```python
from build123d import *

# Parameters (mm, degrees)
SKETCH_1_W               = 135
SKETCH_1_H               = 100
EXTRUDE_1_DEPTH          = 4
SKETCH_2_W               = 135
SKETCH_2_H               = 4
EXTRUDE_2_DEPTH          = 60
CUT_EXTRUDE_1_DEPTH      = 130.12106722
CUT_EXTRUDE_1_DEPTH_BACK = 130.12106722
SKETCH_3_W               = 3
SKETCH_3_H               = 50
FILLET_1_R               = 5
FILLET_2_R               = 2
CUT_EXTRUDE_2_DEPTH      = 130.12106722
CUT_EXTRUDE_2_DEPTH_BACK = 130.12106722
SKETCH_4_R               = 1.75
CUT_EXTRUDE_3_DEPTH      = 130.12106722
CUT_EXTRUDE_3_DEPTH_BACK = 130.12106722
SKETCH_5_W               = 34
SKETCH_5_H               = 12
CUT_EXTRUDE_4_DEPTH      = 130.12106722
CUT_EXTRUDE_4_DEPTH_BACK = 130.12106722
SKETCH_6_R               = 1.75
CUT_EXTRUDE_5_DEPTH      = 130.12106722
CUT_EXTRUDE_5_DEPTH_BACK = 130.12106722
SKETCH_7_R               = 1.63491013
CUT_EXTRUDE_6_DEPTH      = 130.12106722
CUT_EXTRUDE_6_DEPTH_BACK = 130.12106722
SKETCH_8_R               = 1.5
SKETCH_9_R               = 1.75
EXTRUDE_3_DEPTH          = 3
CUT_EXTRUDE_7_DEPTH      = 130.12106722
CUT_EXTRUDE_7_DEPTH_BACK = 130.12106722
SKETCH_10_R              = 1.75


with BuildPart() as part:
    # 草图1 → 凸台-拉伸1 (new body)
    with BuildSketch(Plane(origin=(0, 0, 0), x_dir=(1, 0, 0), z_dir=(0, 1, 0))):
        Rectangle(SKETCH_1_W, SKETCH_1_H)
    extrude(amount=EXTRUDE_1_DEPTH)

    # 草图2 → 凸台-拉伸2 (add)
    with BuildSketch(Plane.XY.offset(50)):
        with Locations((0, 2)):
            Rectangle(SKETCH_2_W, SKETCH_2_H)
    extrude(amount=EXTRUDE_2_DEPTH)

    # 草图3 → 切除-拉伸1 (cut, two sides: drawn at the far end of the back side and taken through both)
    with BuildSketch(Plane(origin=(0, 4, 0), x_dir=(1, 0, 0), z_dir=(0, 1, 0)).offset(-CUT_EXTRUDE_1_DEPTH_BACK)):
        with Locations((-66, 25)):
            Rectangle(SKETCH_3_W, SKETCH_3_H)
        with Locations((66, 25)):
            Rectangle(SKETCH_3_W, SKETCH_3_H)
        with Locations((-66, -85)):
            Rectangle(SKETCH_3_W, SKETCH_3_H)
        with Locations((66, -85)):
            Rectangle(SKETCH_3_W, SKETCH_3_H)
    extrude(amount=CUT_EXTRUDE_1_DEPTH + CUT_EXTRUDE_1_DEPTH_BACK, mode=Mode.SUBTRACT)

    # 圆角1
    fillet_1_edges = [part.edges().sort_by_distance(p)[0] for p in [
        (64.5, 2, -50),
        (-64.5, 2, 110),
        (64.5, 2, 110),
        (-64.5, 2, -50),
    ]]
    fillet(fillet_1_edges, radius=FILLET_1_R)

    # 圆角2
    fillet_2_edges = [part.edges().sort_by_distance(p)[0] for p in [
        (67.5, 2, 0),
        (-67.5, 2, 60),
        (67.5, 2, 60),
        (-67.5, 2, 0),
    ]]
    fillet(fillet_2_edges, radius=FILLET_2_R)

    # 草图4 → 切除-拉伸2 (cut, two sides: drawn at the far end of the back side and taken through both)
    with BuildSketch(Plane(origin=(0, 4, 0), x_dir=(1, 0, 0), z_dir=(0, 1, 0)).offset(-CUT_EXTRUDE_2_DEPTH_BACK)):
        with Locations(Location((-30, -102, 0), (0, 0, 270))):
            Circle(SKETCH_4_R)
        with Locations(Location((0, -102, 0), (0, 0, 270))):
            Circle(SKETCH_4_R)
        with Locations(Location((30, -102, 0), (0, 0, 270))):
            Circle(SKETCH_4_R)
        with Locations(Location((-30, 42, 0), (0, 0, 270))):
            Circle(SKETCH_4_R)
        with Locations(Location((0, 42, 0), (0, 0, 270))):
            Circle(SKETCH_4_R)
        with Locations(Location((30, 42, 0), (0, 0, 270))):
            Circle(SKETCH_4_R)
    extrude(amount=CUT_EXTRUDE_2_DEPTH + CUT_EXTRUDE_2_DEPTH_BACK, mode=Mode.SUBTRACT)

    # 草图5 → 切除-拉伸3 (cut, two sides: drawn at the far end of the back side and taken through both)
    with BuildSketch(Plane(origin=(0, 4, 0), x_dir=(1, 0, 0), z_dir=(0, 1, 0)).offset(-CUT_EXTRUDE_3_DEPTH_BACK)):
        with Locations((0, -86)):
            Rectangle(SKETCH_5_W, SKETCH_5_H)
        with Locations((0, 26)):
            Rectangle(SKETCH_5_W, SKETCH_5_H)
    extrude(amount=CUT_EXTRUDE_3_DEPTH + CUT_EXTRUDE_3_DEPTH_BACK, mode=Mode.SUBTRACT)

    # 草图6 → 切除-拉伸4 (cut, two sides: drawn at the far end of the back side and taken through both)
    with BuildSketch(Plane.XZ.offset(-CUT_EXTRUDE_4_DEPTH_BACK)):
        with Locations(Location((-16, -2, 0), (0, 0, 270))):
            Circle(SKETCH_6_R)
        with Locations(Location((16, -2, 0), (0, 0, 270))):
            Circle(SKETCH_6_R)
        with Locations(Location((16, 62, 0), (0, 0, 270))):
            Circle(SKETCH_6_R)
        with Locations(Location((-16, 62, 0), (0, 0, 270))):
            Circle(SKETCH_6_R)
    extrude(amount=CUT_EXTRUDE_4_DEPTH + CUT_EXTRUDE_4_DEPTH_BACK, mode=Mode.SUBTRACT)

    # 草图7 → 切除-拉伸5 (cut, two sides: drawn at the far end of the back side and taken through both)
    with BuildSketch(Plane.XZ.offset(-CUT_EXTRUDE_5_DEPTH_BACK)):
        with Locations(Location((18, 30.7, 0), (0, 0, 270))):
            Circle(SKETCH_7_R)
        with Locations(Location((-18, 30.7, 0), (0, 0, 270))):
            Circle(SKETCH_7_R)
    extrude(amount=CUT_EXTRUDE_5_DEPTH + CUT_EXTRUDE_5_DEPTH_BACK, mode=Mode.SUBTRACT)

    # 草图8 → 切除-拉伸6 (cut, two sides: drawn at the far end of the back side and taken through both)
    with BuildSketch(Plane.XZ.offset(-CUT_EXTRUDE_6_DEPTH_BACK)):
        with Locations(Location((-41.861200423, 2.110999836, 0), (0, 0, 270))):
            Circle(SKETCH_8_R)
        with Locations(Location((-41.861200325, -46.885600164, 0), (0, 0, 270))):
            Circle(SKETCH_8_R)
        with Locations(Location((16.138810577, 2.110999952, 0), (0, 0, 270))):
            Circle(SKETCH_8_R)
        with Locations(Location((16.138810675, -46.885600048, 0), (0, 0, 270))):
            Circle(SKETCH_8_R)
    extrude(amount=CUT_EXTRUDE_6_DEPTH + CUT_EXTRUDE_6_DEPTH_BACK, mode=Mode.SUBTRACT)

    # 草图9 → 凸台-拉伸3 (add)
    with BuildSketch(Plane.XZ):
        with Locations(Location((16, -2, 0), (0, 0, 270))):
            Circle(SKETCH_9_R)
    extrude(amount=-EXTRUDE_3_DEPTH)

    # 草图10 → 切除-拉伸7 (cut, two sides: drawn at the far end of the back side and taken through both)
    with BuildSketch(Plane(origin=(0, 4, 0), x_dir=(1, 0, 0), z_dir=(0, 1, 0)).offset(-CUT_EXTRUDE_7_DEPTH_BACK)):
        with Locations(Location((63, -10, 0), (0, 0, 270))):
            Circle(SKETCH_10_R)
        with Locations(Location((63, -20, 0), (0, 0, 270))):
            Circle(SKETCH_10_R)
        with Locations(Location((63, -30, 0), (0, 0, 270))):
            Circle(SKETCH_10_R)
        with Locations(Location((63, -40, 0), (0, 0, 270))):
            Circle(SKETCH_10_R)
        with Locations(Location((63, -50, 0), (0, 0, 270))):
            Circle(SKETCH_10_R)
        with Locations(Location((-63, -10, 0), (0, 0, 270))):
            Circle(SKETCH_10_R)
        with Locations(Location((-63, -20, 0), (0, 0, 270))):
            Circle(SKETCH_10_R)
        with Locations(Location((-63, -30, 0), (0, 0, 270))):
            Circle(SKETCH_10_R)
        with Locations(Location((-63, -40, 0), (0, 0, 270))):
            Circle(SKETCH_10_R)
        with Locations(Location((-63, -50, 0), (0, 0, 270))):
            Circle(SKETCH_10_R)
    extrude(amount=CUT_EXTRUDE_7_DEPTH + CUT_EXTRUDE_7_DEPTH_BACK, mode=Mode.SUBTRACT)


solid = part.part
```
Read the model definition and answer for the solid it produces. Units are mm, in the model's axes. A direction names the side the tool comes from. Give positions to 0.01 mm unless a question says otherwise; leave off trailing zeros. Write each loop counter-clockwise with the first axis right and the second up, starting at its lowest first coordinate (ties: lowest second). Pieces come first, ordered by that corner, then holes. Notation, with made-up numbers: (79.5, 30) - (116.5, 30) arc R26 ccw to (116.5, 56) - close; hole circle Ø4 at (32, -3.75). An arc over 180 degrees is marked (long way). Write item = value, one per line. Start each with the question number.
Item 1: The mould has two halves that part along X. Classify faces 4 (the flat face through (-1, 2, -50)), 5 (the cylindrical face through (-63.07, 2.03, 108.5)), 6 (the cylindrical face through (-64.71, 1.97, 29.62)): +X half, -X half, draft (parallel to the pull), parting line (faces both ways), or undercut.
Item 2: Each of these flat-tipped pins is pushed along its axis until it touches: P1, Ø0.8, axis at x = 65, y = 2.5, coming from the +Z side; P2, Ø0.8, axis at x = -65, y = 1.5, coming from the -Z side; P3, Ø2, axis at y = 1.5, z = -26, coming from the -X side. Where does it stop, or does it pass through?
Item 3: Find section D-D (z = -2). Give the vertices of the cut face in (x, y).
Item 4: A tool of negligible diameter and unlimited length cuts with its end or side. For faces 1 (the flat face through (64.5, 2, 83)), 2 (the flat face through (0, 2, -32)), 3 (the cylindrical face through (17.735, 3.507, -1.772)), from which of +Z, -Z, +X, -X, +Y, -Y can it reach the whole face along a straight path? Write none if from no direction.
Item 5: Find section B-B (z = 50). Give the vertices of the cut face in (x, y).
Item 6: Find section A-A (z = -42). Give the vertices of the cut face in (x, y).
Item 7: Find the intervals of material crossed by probe 1 along Z at (x, y) = (30, 3.05); probe 2 along X at (y, z) = (2.15, 10); probe 3 along Z at (x, y) = (-16, 1.2), in increasing order. Write a range as [from, to].
Item 8: Find section C-C (x = 0). Give the vertices of the cut face in (y, z).
Response:
q1.face_4 = draft
q1.face_5 = -X half
q1.face_6 = undercut
q2.P1 = 60
q2.P2 = 0
q2.P3 = -64.5
q3.outline = (-64.5, 0) - (-17.75, 0) - (-17.75, 4) - (-64.5, 4) - close; (-14.25, 0) - (64.5, 0) - (64.5, 4) - (17.75, 4) - (17.75, 3) - (14.25, 3) - (14.25, 4) - (-14.25, 4) - close
q4.face_1 = +Z, +X, +Y, -Y
q4.face_2 = +Y, -Y
q4.face_3 = +Y
q5.outline = (-67.5, 0) - (-64.75, 0) - (-64.75, 4) - (-67.5, 4) - close; (-61.25, 0) - (61.25, 0) - (61.25, 4) - (-61.25, 4) - close; (64.75, 0) - (67.5, 0) - (67.5, 4) - (64.75, 4) - close
q6.outline = (-64.5, 0) - (-31.75, 0) - (-31.75, 4) - (-64.5, 4) - close; (-28.25, 0) - (-1.75, 0) - (-1.75, 4) - (-28.25, 4) - close; (1.75, 0) - (28.25, 0) - (28.25, 4) - (1.75, 4) - close; (31.75, 0) - (64.5, 0) - (64.5, 4) - (31.75, 4) - close
q7.probe_1 = [-50, -43.75], [-40.25, 100.25], [103.75, 110]
q7.probe_2 = [-67.5, -64.75], [-61.25, 61.25], [64.75, 67.5]
q7.probe_3 = [-50, -32], [-20, -3.75], [-0.25, 60.25], [63.75, 80], [92, 110]
q8.outline = (0, -50) - (4, -50) - (4, -43.75) - (0, -43.75) - close; (0, -40.25) - (4, -40.25) - (4, -32) - (0, -32) - close; (0, -20) - (4, -20) - (4, 80) - (0, 80) - close; (0, 92) - (4, 92) - (4, 100.25) - (0, 100.25) - close; (0, 103.75) - (4, 103.75) - (4, 110) - (0, 110) - close
